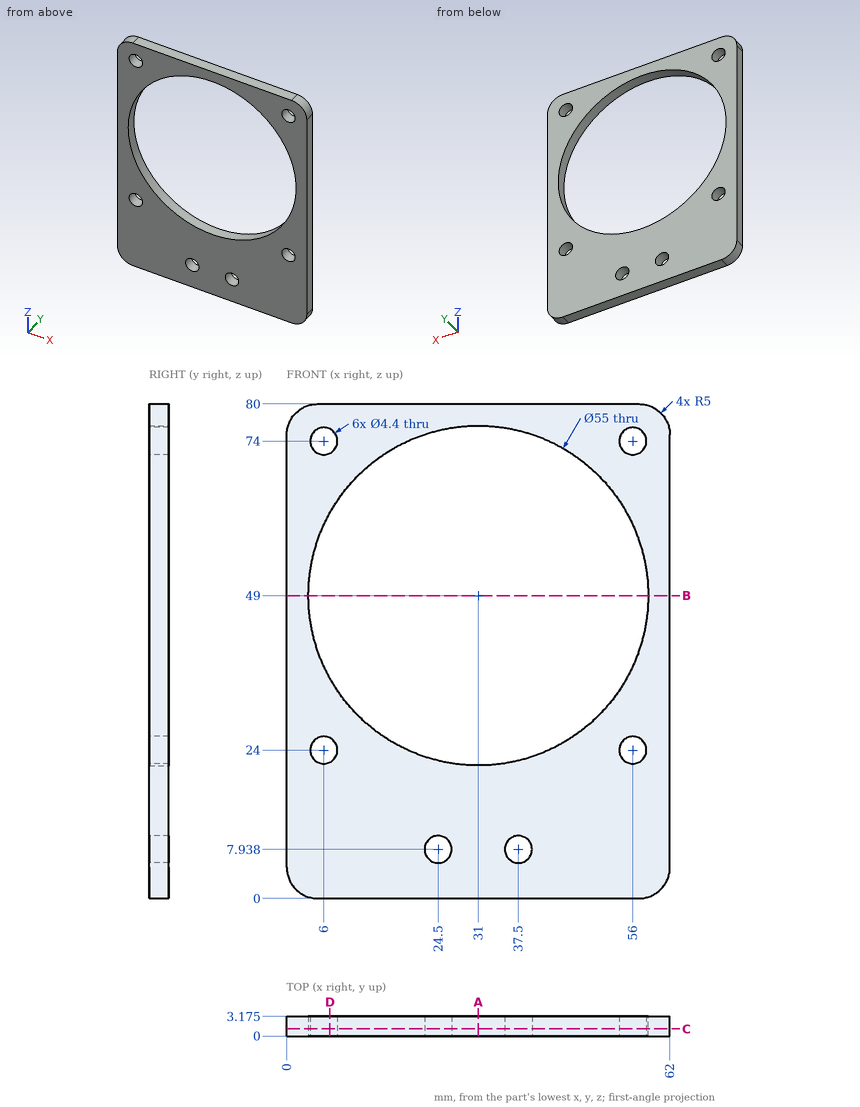
Can you work these out from the drawing? Everything is in mm from the part's minimum corner. Coordinates: 2 decimals unless noted, no trailing zeros. Write each loop counter-clockwise with the first axis right and the second up, starting at its lowest first coordinate (ties: lowest second). Pieces come first, ordered by that corner, then holes. Notation, with made-up numbers: (2, 4) -> (20, 4) arc R18 cw to (20, 23) -> close; hole circle Ø3 at (51.25, 23). An arc over 180 degrees is marked (long way). Return JSON: item names as keys, results as strings.
(1) Imagine slicing it at D-D, the plane x = 7. Please give me the cut outline in (y, z) (1 decimal), then the cut area to 3 significant figures.
Numbers:
{"outline": "(0, 0) -> (3.2, 0) -> (3.2, 22) -> (0, 22) -> close; (0, 26) -> (3.2, 26) -> (3.2, 35.6) -> (0, 35.6) -> close; (0, 62.4) -> (3.2, 62.4) -> (3.2, 72) -> (0, 72) -> close; (0, 76) -> (3.2, 76) -> (3.2, 80) -> (0, 80) -> close", "area": "144 mm2"}
(2) Imagine slicing it at A-A, the plane x = 31. Please give me the cut outline in (y, z) (1 decimal).
Numbers:
{"outline": "(0, 0) -> (3.2, 0) -> (3.2, 21.5) -> (0, 21.5) -> close; (0, 76.5) -> (3.2, 76.5) -> (3.2, 80) -> (0, 80) -> close"}
(3) I need wall thicknesses on L1, parallel to Z at x = 56, y = 1.55 (1 decimal); L2, parallel to X at y = 2.4, z = 25.5 (1 decimal); L3, parallel to Z at x = 24.5, y = 1.6. Which ranges of each line are inside material? Lowest first, please.
Numbers:
{"L1": "z = 0 to 21.8, 26.2 to 37.5, 60.5 to 71.8, 76.2 to 80", "L2": "x = 0 to 4.4, 7.6 to 16.7, 45.3 to 54.4, 57.6 to 62", "L3": "z = 0 to 5.74, 10.14 to 22.28, 75.72 to 80"}
(4) Imagine slicing it at C-C, the plane y = 1.15. Please give me the cut outline in (x, z), then the cut area to 3 significant figures.
Numbers:
{"outline": "(0, 5) arc R5 ccw to (5, 0) -> (57, 0) arc R5 ccw to (62, 5) -> (62, 75) arc R5 ccw to (57, 80) -> (5, 80) arc R5 ccw to (0, 75) -> close; hole circle Ø55 at (31, 49); hole circle Ø4.4 at (6, 24); hole circle Ø4.4 at (6, 74); hole circle Ø4.4 at (24.5, 7.94); hole circle Ø4.4 at (37.5, 7.94); hole circle Ø4.4 at (56, 24); hole circle Ø4.4 at (56, 74)", "area": "2,470 mm2"}
(5) Imagine slicing it at B-B, the plane z = 49. Please give me the cut outline in (x, y) (1 decimal).
Numbers:
{"outline": "(0, 0) -> (3.5, 0) -> (3.5, 3.2) -> (0, 3.2) -> close; (58.5, 0) -> (62, 0) -> (62, 3.2) -> (58.5, 3.2) -> close"}
